Build history of the part. All positions in model axes, mm. Round coordinates to 2 decimals unless told otherwise and drop trailing zeros. Order: outer loops, then holes, each group sorted by start corner. A loop starts at its lowest first (then second) coordinate and runs counter-clockwise, first axis right, second up. Notation, with made-up numbers: (-11, 20.25) -> (26, 20.25) arc R24 cw to (26, 40.25) -> close; hole circle Ø7 at (-35.75, 85.25). An arc over 180 degrees is marked (long way). Answer as a JSON object with one key per item and string values.
from build123d import *

# Parameters (mm, degrees)
SKETCH1_W           = 139.5
SKETCH1_H           = 152.4
BOSS_EXTRUDE1_DEPTH = 6.35
SKETCH2_W           = 6.35
SKETCH2_H           = 152.4
CUT_EXTRUDE1_DEPTH  = 3.375
SKETCH3_R           = 7.62
SKETCH3_W           = 15.24
SKETCH3_H           = 12.7
CUT_EXTRUDE2_DEPTH  = 7.35


with BuildPart() as part:
    # Sketch1 → Boss-Extrude1 (new body)
    with BuildSketch(Plane(origin=(0, 0, 0), x_dir=(1, 0, 0), z_dir=(0, 1, 0))):
        with Locations((69.75, 76.2)):
            Rectangle(SKETCH1_W, SKETCH1_H)
    extrude(amount=BOSS_EXTRUDE1_DEPTH)

    # Sketch2 → Cut-Extrude1 (cut)
    with BuildSketch(Plane(origin=(0, 6.35, 0), x_dir=(1, 0, 0), z_dir=(0, 1, 0))):
        with Locations((3.175, 76.2)):
            Rectangle(SKETCH2_W, SKETCH2_H)
        with Locations((136.325, 76.2)):
            Rectangle(SKETCH2_W, SKETCH2_H)
    extrude(amount=-CUT_EXTRUDE1_DEPTH, mode=Mode.SUBTRACT)

    # Sketch3 → Cut-Extrude2 (cut, through all)
    with BuildSketch(Plane(origin=(0, 6.35, 0), x_dir=(1, 0, 0), z_dir=(0, 1, 0))):
        with Locations((62.892, 31.75)):
            Circle(SKETCH3_R)
        with Locations((69.75, 6.35)):
            Rectangle(SKETCH3_W, SKETCH3_H)
    extrude(amount=-CUT_EXTRUDE2_DEPTH, mode=Mode.SUBTRACT)


solid = part.part
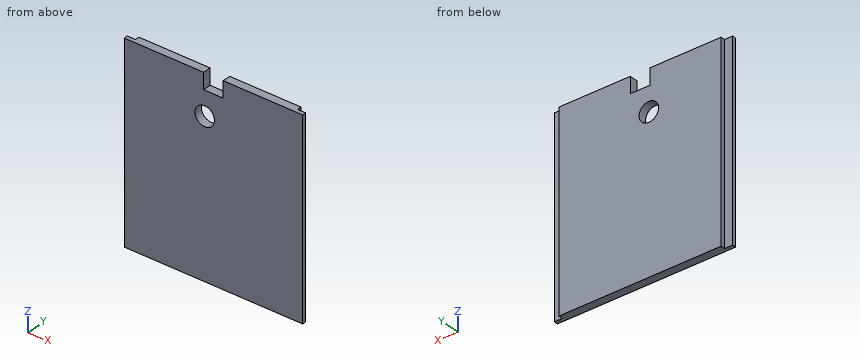
1) Flat gauge pins, fed straight in: pin 1 Ø1 at (y, z) = (4, -63.5) entering from +X; pin 2 Ø1.9 at (x, z) = (3, -113) entering from +Y (3 decimals); pin 3 Ø1 at (y, z) = (4, -97) entering from -X. Where does each tip first touch, or does it go through?
Checked values:
{"pin 1": "stops at x = 133.15", "pin 2": "stops at y = 2.975", "pin 3": "stops at x = 6.35"}
2) Probe L1, parallel to X at y = 2.25, z = -31.75; L2, parallel to X at y = 4.5, z = -31.75; L3, parallel to Z at x = 56, y = 5.75. List the from-to ranges inside material, lowest first. Write a range as from..to.
Checked values:
{"L1": "x = 0..55.27, 70.51..139.5", "L2": "x = 6.35..55.27, 70.51..133.15", "L3": "z = -152.4..-35, -28.5..0"}
3) Cut at A-A, the plane z = -31.75. Give the cut face in (x, y) (3 decimals).
Checked values:
{"outline": "(0, 0) -> (55.272, 0) -> (55.272, 6.35) -> (6.35, 6.35) -> (6.35, 2.975) -> (0, 2.975) -> close; (70.512, 0) -> (139.5, 0) -> (139.5, 2.975) -> (133.15, 2.975) -> (133.15, 6.35) -> (70.512, 6.35) -> close"}
